```python
from build123d import *

# Parameters (mm, degrees)
BOSS_EXTRUDE3_DEPTH = 50.5
SKETCH6_R           = 20
BOSS_EXTRUDE4_DEPTH = 26
SKETCH7_R           = 10
CUT_EXTRUDE1_DEPTH  = 26
CUT_EXTRUDE2_DEPTH  = 19


with BuildPart() as part:
    # Sketch4 → Boss-Extrude3 (new body)
    with BuildSketch(Plane(origin=(0, 0, 0), x_dir=(1, 0, 0), z_dir=(0, 1, 0))):
        Polygon((0, 0), (70, 0), (85, 34), (85, 50), (57.5, 50), (47, 19), (23, 19), (12.5, 50), (-15, 50), (-15, 34), align=None)
    extrude(amount=BOSS_EXTRUDE3_DEPTH)

    # Sketch6 → Boss-Extrude4 (add)
    with BuildSketch(Plane.XY):
        with Locations(Location((35, 25.25, 0), (0, 0, 180))):
            Circle(SKETCH6_R)
    extrude(amount=BOSS_EXTRUDE4_DEPTH)

    # Sketch7 → Cut-Extrude1 (cut)
    with BuildSketch(Plane.XY.offset(26)):
        with Locations((35, 25.25)):
            Circle(SKETCH7_R)
    extrude(amount=-CUT_EXTRUDE1_DEPTH, mode=Mode.SUBTRACT)

    # Sketch8 → Cut-Extrude2 (cut)
    with BuildSketch(Plane.XY):
        Polygon((80, 25.855466689), (80, 35.25), (60, 35.25), (60, 15.25), (80, 15.25), align=None)
        Polygon((-10, 25.855466689), (-10, 35.25), (10, 35.25), (10, 15.25), (-10, 15.25), align=None)
    extrude(amount=-CUT_EXTRUDE2_DEPTH, mode=Mode.SUBTRACT)


solid = part.part
```
Can you work these out from the model? Positions are in its coordinate system, mm. A direction names the side the tool comes from. Give positions to 0.01 mm unless a question says otherwise; leave off trailing zeros. Order: outer loops, then holes, each group sorted by start corner. A loop starts at its lowest first (then second) coordinate and runs counter-clockwise, first axis right, second up. Notation, with made-up numbers: M 37.5,25 L 57.5,25 A37 cw 57.5,64 Z; hole C 39,29 d5. An arc over 180 degrees is marked long. One line per item, written item: value.
1) I want a section at B-B, the plane z = -30.5. List the corners of the cut face in (x, y) for me.
Answer sheet:
outline: M -13.46,0 L 19.1,0 L 19.1,50.5 L -13.46,50.5 Z; M 50.9,0 L 83.46,0 L 83.46,50.5 L 50.9,50.5 Z
2) Please list where these lines run through material, in increasing order: line 1 along Y through (x, z) = (35, 7.25); line 2 along X through (y, z) = (25, 15); line 3 along Z through (x, y) = (32, 18).
Answer sheet:
line 1: y = 5.25 to 15.25, 35.25 to 45.25
line 2: x = 15 to 25, 45 to 55
line 3: z = -19 to 0
3) On a 3-axis mill with a long thin cutter (end or side, diameter ignored), from which of +Z, -Z, +X, -X, +Y, -Y can I reach the whole of each face in a straight line? I mean faces 5 (the face through (69, 25, -19)), 6 (the face through (35, 25, -19)), 7 (the face through (35, 25, 0)), 8 (the face through (40, 16, 26)), 9 (the face through (3, 15.25, -9)). Say none if no direction works.
Answer sheet:
face 5: +Z, +X
face 6: -Z, +Y, -Y
face 7: +Z
face 8: +Z, +X, -X, +Y, -Y
face 9: +Z, -X
4) I want a section at C-C, the plane y = 25.25. List the corners of the cut face in (x, z) for me, plus the area to 3 significant figures.
Answer sheet:
outline: M -15,-50 L 12.5,-50 L 23,-19 L 47,-19 L 57.5,-50 L 85,-50 L 85,-34 L 78.38,-19 L 60,-19 L 60,0 L 55,0 L 55,26 L 45,26 L 45,0 L 25,0 L 25,26 L 15,26 L 15,0 L 10,0 L 10,-19 L -8.38,-19 L -15,-34 Z
area: 3,400 mm^2
5) We'd pull the mould along X, two halves only. Please class faces 1 (the face through (-9.272, 24.896, -21.016)), 2 (the face through (85, 25, -42)), 3 (the face through (17.824, 24.896, -34.283)), 4 (the face through (52.323, 24.896, -34.717)): released by +X, released by -X, zero draft, split by the parting line, or undercut.
Answer sheet:
face 1: released by -X
face 2: released by +X
face 3: undercut
face 4: undercut
6) For P1, Ø15, axis at y = 27.5, z = -8, coming from the -X side; P2, Ø20, axis at x = -1, y = 25, coming from the +Z side; P3, Ø3, axis at y = 8.5, z = -16, coming from the +X side, each with a flat end and sliding along its axis, tell me the tip position at first contact or that it passes through.
Answer sheet:
P1: stops at x = 10
P2: stops at z = 0
P3: stops at x = 77.72
7) I want a section at D-D, the plane z = 9. List the corners of the cut face in (x, y) for me, plus the area to 3 significant figures.
Answer sheet:
outline: C 35,25.25 d40; hole C 35,25.25 d20
area: 942 mm^2
8) I want a section at A-A, the plane x = 35. List the corners of the cut face in (y, z) for me, plus the area to 3 significant figures.
Answer sheet:
outline: M 0,-19 L 50.5,-19 L 50.5,0 L 45.25,0 L 45.25,26 L 35.25,26 L 35.25,0 L 15.25,0 L 15.25,26 L 5.25,26 L 5.25,0 L 0,0 Z
area: 1,480 mm^2
